Read the model definition and answer for the solid it produces. Units are mm, in the model's axes. Face numbers are marked on the shaded views. A direction names the side the tool comes from. Coordinates: 2 decimals unless noted, no trailing zeros. Write each loop counter-clockwise with the first axis right and the second up, starting at its lowest first coordinate (ties: lowest second). Pieces come first, ordered by that corner, then holes. Notation, with made-up numbers: (88, 66) -> (125, 66) arc R27 ccw to (125, 97) -> close; hole circle Ø1 at (4, 0.25). An arc over 180 degrees is marked (long way). One line per item, written item: value. Start each with the question number.
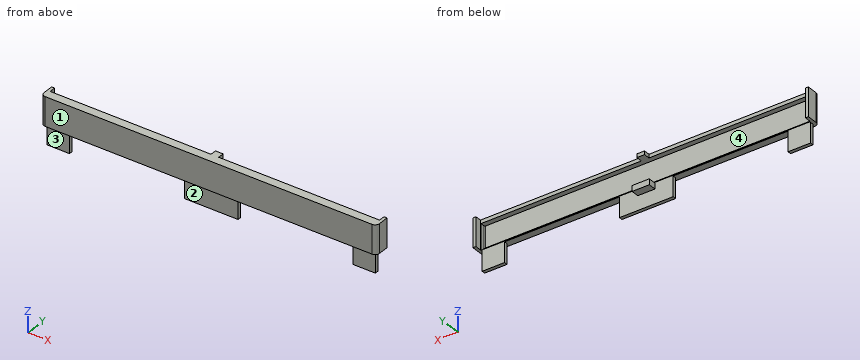
Solid Edge part; units mm, degrees
sketch "Sketch1" plane through (-62.4275, 25.9494, 0) normal (0, 0, 1) x (-1, 0, 0)
  line L0 (75.064, 25.4416) -> (75.064, 28.4894)
  line L1 (75.064, 30.1404) -> (75.064, 28.4894)
  arc A0 (73.159, 32.0454) -> (75.064, 30.1404) centre (73.159, 30.1404) cw
  line L2 (-71.889, 32.0454) -> (73.159, 32.0454)
  arc A1 (-73.794, 30.1404) -> (-71.889, 32.0454) centre (-71.889, 30.1404) cw
  line L3 (-73.794, 28.4894) -> (-73.794, 30.1404)
  line L4 (-73.794, 28.4894) -> (-73.794, 25.4416)
  line L5 (-73.794, 25.4416) -> (-72.2065, 25.4416)
  line L6 (-72.2065, 26.9019) -> (-72.2065, 25.4416)
  line L7 (-72.2065, 26.9019) -> (-72.2065, 30.1404)
  arc A2 (-72.2065, 30.1404) -> (-71.889, 30.4579) centre (-71.889, 30.1404) cw
  line L8 (-71.889, 30.4579) -> (73.159, 30.4579)
  arc A3 (73.159, 30.4579) -> (73.4765, 30.1404) centre (73.159, 30.1404) cw
  line L9 (73.4765, 30.1404) -> (73.4765, 26.9019)
  line L10 (73.4765, 25.4416) -> (73.4765, 26.9019)
  line L11 (73.4765, 25.4416) -> (75.064, 25.4416)
extrude "Protrusion1" add sketch "Sketch1" along normal up to vertex (12 mm away)
sketch "Sketch2" plane through (-62.4275, -3.81, 12) normal (0, 0, 1) x (-1, 0, 0)
  line L0 (75.064, -4.3178) -> (75.064, 0.381)
  arc A0 (75.064, 0.381) -> (73.159, 2.286) centre (73.159, 0.381) ccw
  line L1 (73.159, 2.286) -> (-71.889, 2.286)
  arc A1 (-71.889, 2.286) -> (-73.794, 0.381) centre (-71.889, 0.381) ccw
  line L2 (-73.794, -1.27) -> (-73.794, 0.381)
  line L3 (-73.794, -1.27) -> (-73.794, -4.3178)
  line L4 (75.064, -4.3178) -> (-73.794, -4.3178)
extrude "Protrusion2" add sketch "Sketch2" along normal mid plane 1.5875
sketch "Sketch3" plane through (-62.4275, -3.81, 12.7938) normal (0, 0, 1) x (-1, 0, 0)
  line L0 (73.7432, -1.5748) -> (73.7432, -63.278)
  line L1 (73.7432, -63.278) -> (2.3368, -63.278)
  line L2 (2.3368, -63.278) -> (2.3368, -1.5748)
  line L3 (2.3368, -1.5748) -> (73.7432, -1.5748)
  line L4 (-72.4732, -63.278) -> (-72.4732, -1.5748)
  line L5 (-72.4732, -1.5748) -> (-1.0668, -1.5748)
  line L6 (-1.0668, -1.5748) -> (-1.0668, -63.278)
  line L7 (-1.0668, -63.278) -> (-72.4732, -63.278)
extrude "Cutout1" cut sketch "Sketch3" against normal up to vertex (12.7938 mm away)
sketch "Sketch4" plane through (-62.4275, -2.7941, 0) normal (0, 0, -1) x (-1, 0, 0)
  line L0 (73.4765, -0.1904) -> (-72.2065, -0.1904)
  line L1 (-72.2065, -0.1904) -> (-72.2065, -1.7144)
  line L2 (-72.2065, -1.7144) -> (73.4765, -1.7144)
  line L3 (73.4765, -0.1904) -> (73.4765, -1.7144)
extrude "ExtrudedProtrusion_3" add sketch "Sketch4" against normal blind 1.5875 and the other way blind 8.89
chamfer "Chamfer_1" distance 1.27 angle 45 1 edges at (-63.0625, -2.9845, 1.5875)
sketch "Sketch5" plane through (-62.4275, -2.7941, 0) normal (0, 0, -1) x (-1, 0, 0)
  line L0 (-3.175, -1.7144) -> (-3.175, 3.3019)
  line L1 (-3.175, 3.3019) -> (4.445, 3.3019)
  line L2 (4.445, 3.3019) -> (4.445, -1.7144)
  line L3 (4.445, -1.7144) -> (-3.175, -1.7144)
extrude "ExtrudedProtrusion_4" add sketch "Sketch5" along normal blind 2.54
sketch "Sketch6" plane through (-62.4275, -4.5085, -4.445) normal (0, -1, 0) x (1, 0, 0)
  line L0 (11.27, -20.066) -> (62.27, -20.066)
  line L1 (62.27, -20.066) -> (62.27, 4.445)
  line L2 (62.27, 4.445) -> (11.27, 4.445)
  line L3 (11.27, 4.445) -> (11.27, -20.066)
  line L4 (-63.54, -20.066) -> (-12.54, -20.066)
  line L5 (-12.54, -20.066) -> (-12.54, 4.445)
  line L6 (-12.54, 4.445) -> (-63.54, 4.445)
  line L7 (-63.54, 4.445) -> (-63.54, -20.066)
extrude "Cutout2" cut sketch "Sketch6" against normal through all
1. A cutting plane is placed at C-C on x = -52.5. Give the vertices of the cut face in (y, z).
2. Find the intervals of material crossed by probe 1 along X at (y, z) = (-2.5, 2.75); probe 2 along X at (y, z) = (0, 7.5); probe 3 along Y at (x, z) = (4.5, 7), in increasing order. Write a range as from..to.
3. A cutting plane is placed at B-B on y = -1. Give the vertices of the cut face in (x, z), then the cut area to 3 significant figures.
4. A tool of negligible diameter and unlimited length cuts with its end or side. For the marked faces 1 and 2, from which of +Z, -Z, +X, -X, +Y, -Y can it reach the whole face along a straight path? Write none if from no direction.
5. Given pin 1 (4.5 mm diameter, centred on x = -66.5, z = -5, fed in from -Y); pin 2 (0.8 mm diameter, centred on y = -3.5, z = -4.5, fed in from -X); pin 3 (2 mm diameter, centred on x = -43, z = 5, fed in from +Y), each flat-ended and moving along its own axis, determine where each tip first touches the part or whether it passes through.
6. A cutting plane is placed at A-A on z = -4.5. Give the vertices of the cut face in (x, y), then the cut area to 3 significant figures.
7. For a pull along Z with two mould halves and no side action, classify the marked faces 3 and 4 as +Z half, -Z half, draft (parallel to the pull), parting line (faces both ways), or undercut.
Derived:
1. outline: (-6.1, 0) -> (-4.51, 0) -> (-4.51, -8.89) -> (-2.98, -8.89) -> (-2.98, 0.32) -> (-4.25, 1.59) -> (-4.51, 1.59) -> (-4.51, 11.21) -> (-2.24, 11.21) -> (-2.24, 12.79) -> (-6.1, 12.79) -> close
2. probe 1: x = -137.49..-135.9, 9.78..11.37
2. probe 2: x = -137.49..-136.17, 10.05..11.37
2. probe 3: y = -6.1..-4.51
3. outline: (-137.49, 0) -> (-136.17, 0) -> (-136.17, 12.79) -> (-137.49, 12.79) -> close; (-66.87, -2.54) -> (-59.25, -2.54) -> (-59.25, 0) -> (-66.87, 0) -> close; (-64.76, 11.21) -> (-61.36, 11.21) -> (-61.36, 12.79) -> (-64.76, 12.79) -> close; (10.05, 0) -> (11.37, 0) -> (11.37, 12.79) -> (10.05, 12.79) -> close
3. area: 58.6 mm2
4. face 1: +Z, -Z, +X, -X, -Y
4. face 2: -Z, +X, -X, -Y
5. pin 1: stops at y = -4.51
5. pin 2: stops at x = -135.9
5. pin 3: stops at y = -4.51
6. outline: (-135.9, -4.51) -> (-125.97, -4.51) -> (-125.97, -2.98) -> (-135.9, -2.98) -> close; (-74.97, -4.51) -> (-51.16, -4.51) -> (-51.16, -2.98) -> (-74.97, -2.98) -> close; (-0.16, -4.51) -> (9.78, -4.51) -> (9.78, -2.98) -> (-0.16, -2.98) -> close
6. area: 66.6 mm2
7. face 3: draft
7. face 4: undercut
